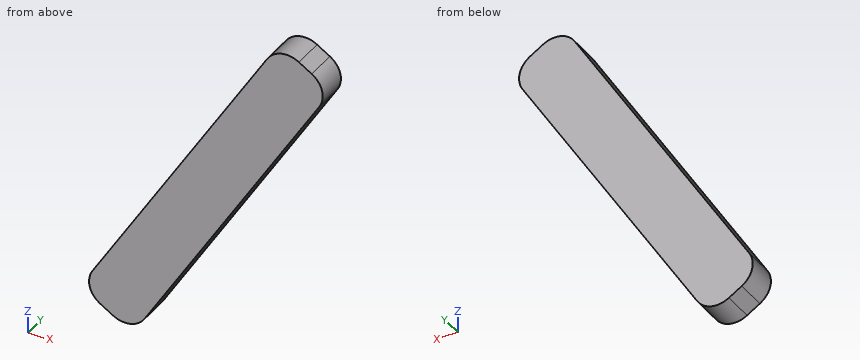
from build123d import *

# Parameters (mm, degrees)
PAD024_DEPTH = 4
FILLET016_R  = 3


with BuildPart() as fillet016:
    # Sketch028 → Pad024 (new body)
    with BuildSketch(Plane.XZ.offset(25)):
        Polygon((-45.702244, -3.721947), (-38.908337, 0.415547), (-12.968213, -41.849118), (-19.76212, -45.986612), align=None)
    extrude(amount=PAD024_DEPTH)

    # Fillet016
    fillet016_edges = [fillet016.edges().sort_by_distance(p)[0] for p in [
        (-45.702244, -27, -3.721947),
        (-38.908337, -27, 0.415547),
        (-12.968213, -27, -41.849118),
        (-19.76212, -27, -45.986612),
    ]]
    fillet(fillet016_edges, radius=FILLET016_R)


with BuildPart() as part_mirroring012:
    # Part__Mirroring012: instance of Fillet016
    add(fillet016.part.mirror(Plane(origin=(0, 0, 0), x_dir=(0, -1, 0), z_dir=(1, 0, 0))))


with BuildPart() as part_mirroring012_1:
    # Part__Mirroring012 placement: moved
    add(part_mirroring012.part.moved(Location((76, 0, 0))))


solid = part_mirroring012_1.part
Design review of the part built by this model. Coordinates are the model's own, in mm. Coordinates: 2 decimals unless noted, no trailing zeros. Order: outer loops, then holes, each group sorted by start corner. A loop starts at its lowest first (then second) coordinate and runs counter-clockwise, first axis right, second up. Notation, with made-up numbers: (-35.75, 8.5) -> (23.25, 8.5) arc R12 ccw to (23.25, 30.5) -> close; hole circle Ø9 at (55, 32). An arc over 180 degrees is marked (long way). Use one line per item in the form item = value. Start each with the question number.
(1) Insertion check: pin 1 (2 mm diameter, centred on y = -27, z = -11.5, fed in from -X); pin 2 (2 mm diameter, centred on x = 117, y = -27, fed in from -Z); pin 3 (1.5 mm diameter, centred on x = 108, y = -28, fed in from +Z). Each pin has a flat end and moves straight along its axis. Give the tip position at first contact, or say it passes through.
(2) Add section B-B on z = -5. State the section outline as (x, y) points.
(3) Add section A-A on y = -26.3. State the section outline as (x, z) points, plus the area to 3 significant figures.
(4) Add section C-C on x = 115. State the section outline as (y, z) points, plus the area to 3 significant figures.
(5) For probe 1 along Z at (x, y) = (112.5, -26.25); probe 2 along X at (y, z) = (-28.65, -7); probe 3 along X at (y, z) = (-25.5, -23), list the stretches that pass through material, from the lowest coordinate up.
Answer block:
q1.pin_1 = 106.98
q1.pin_2 = -13.01
q1.pin_3 = -9.62
q2.outline = (111.58, -29) -> (120.56, -29) -> (120.56, -25) -> (111.58, -25) -> close
q3.outline = (90.54, -39.28) arc R3 ccw to (91.54, -43.41) -> (93.21, -44.43) arc R3 ccw to (97.33, -43.44) -> (120.13, -6.29) arc R3 ccw to (119.13, -2.16) -> (117.46, -1.14) arc R3 ccw to (113.34, -2.13) -> close
q3.area = 387 mm²
q4.outline = (-29, -14.64) -> (-25, -14.64) -> (-25, -0.84) -> (-29, -0.84) -> close
q4.area = 55.2 mm²
q5.probe_1 = -18.72 to -3.51
q5.probe_2 = 110.36 to 119.69
q5.probe_3 = 100.54 to 109.87
